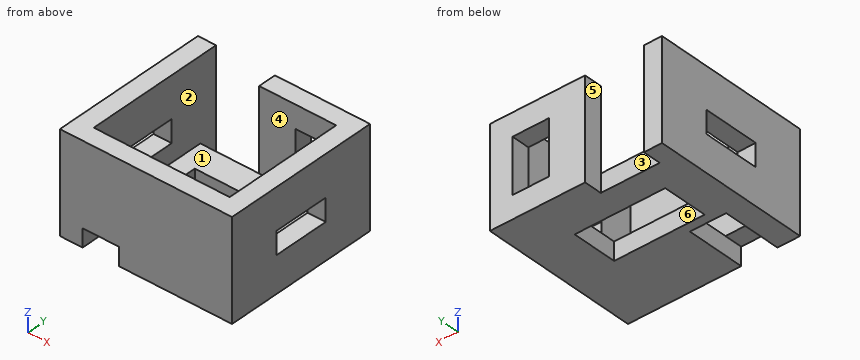
from build123d import *

# Parameters (mm, degrees)
F0_W     = 4
F0_H     = 4
F0_W_2   = 10
F0_H_2   = 5
F1_DEPTH = 2
F2_DEPTH = 11
F3_W     = 4
F3_H     = 6
F4_DEPTH = 2.9
F5_W     = 6.25
F5_H     = 2.5
F6_DEPTH = 20
F7_W     = 4
F7_H     = 2
F8_DEPTH = 2.8


with BuildPart() as f1:
    # F0 (on Top) → F1 (new body)
    with BuildSketch(Plane.XY):
        Polygon((-7.5, -6.75), (7.5, -6.75), (7.5, 6.75), (-1, 6.75), (-7.5, 6.75), align=None)
        with Locations((-5, -4.25)):
            Rectangle(F0_W, F0_H, mode=Mode.SUBTRACT)
        with Locations((-0.5, 1.25)):
            Rectangle(F0_W_2, F0_H_2, mode=Mode.SUBTRACT)
    extrude(amount=F1_DEPTH)

    # F0 (on Top) → F2 (join)
    with BuildSketch(Plane.XY):
        Polygon((7.5, 6.75), (7.5, -6.75), (-7.5, -6.75), (-7.5, 6.75), (-7.5, 8.75), (-9.5, 8.75), (-9.5, -8.75), (9.5, -8.75), (9.5, 8.75), (-1, 8.75), (-1, 6.75), align=None)
    extrude(amount=F2_DEPTH)

    # F3 (on face) → F4 (cut)
    with BuildSketch(Plane(origin=(0, 8.75, 0), x_dir=(-1, 0, 0), z_dir=(0, 1, 0))):
        with Locations((-5, 5.5)):
            Rectangle(F3_W, F3_H)
    extrude(amount=-F4_DEPTH, mode=Mode.SUBTRACT)

    # F5 (on face) → F6 (cut)
    with BuildSketch(Plane.YZ.offset(9.5)):
        with Locations((0, 5.25)):
            Rectangle(F5_W, F5_H)
    extrude(amount=-F6_DEPTH, mode=Mode.SUBTRACT)

    # F7 (on face) → F8 (cut)
    with BuildSketch(Plane.XZ.offset(8.75)):
        with Locations((-5, 1)):
            Rectangle(F7_W, F7_H)
    extrude(amount=-F8_DEPTH, mode=Mode.SUBTRACT)


solid = f1.part
Here's how the part is built. I have some questions about the finished solid (model axes, mm). Face numbers are marked on the shaded views. A direction names the side the tool comes from. Give positions to 0.01 mm unless a question says otherwise; leave off trailing zeros. Order: outer loops, then holes, each group sorted by start corner. A loop starts at its lowest first (then second) coordinate and runs counter-clockwise, first axis right, second up. Notation, with made-up numbers: (31.25, 32.5) -> (84.25, 32.5) arc R24 ccw to (84.25, 46.5) -> close; hole circle Ø11 at (53, 30). An arc over 180 degrees is marked (long way). One line per item, written item: value. Start each with the question number.
1. Imagine slicing it at D-D, the plane y = -1.5. List the corners of the cut face in (x, z) for me.
2. I need wall thicknesses on probe 1 along X at (y, z) = (-6.25, 4.25); probe 2 along Y at (x, z) = (2.25, 2.5); probe 3 along Y at (x, z) = (-4.5, 2.75). Which ranges of each line are inside material? Lowest first, please. Write a range as from..to.
3. Imagine slicing it at A-A, the plane y = -6. List the corners of the cut face in (x, z) for me, plus the area to 3 significant figures.
4. Imagine slicing it at C-C, the plane z = 6.75. List the corners of the cut face in (x, y) for me, plus the area to 3 significant figures.
5. For the marked faces 4, 5 and 6, which set-ups out of +Z, -Z, +X, -X, +Y, -Y let a thin tool reach every point of the face, with its end or its side?
6. Imagine slicing it at B-B, the plane x = 0. List the corners of the cut face in (y, z) for me.
7. Will these pins go through, and if not, where does the flat tip stop? pin 1 Ø5 at (x, y) = (-1.5, 4) entering from -Z; pin 2 Ø1 at (x, y) = (-4.5, -7.5) entering from -Z; pin 3 Ø7 at (x, y) = (2.5, -2.5) entering from +Z.
8. We'd pull the mould along Y, two halves only. Please class the marked faces 1, 2 and 3: released by +Y, released by -Y, zero draft, split by the parting line, or undercut.
Values follow:
1. outline: (-9.5, 0) -> (9.5, 0) -> (9.5, 4) -> (7.5, 4) -> (7.5, 2) -> (-7.5, 2) -> (-7.5, 4) -> (-9.5, 4) -> close; (-9.5, 6.5) -> (-7.5, 6.5) -> (-7.5, 11) -> (-9.5, 11) -> close; (7.5, 6.5) -> (9.5, 6.5) -> (9.5, 11) -> (7.5, 11) -> close
2. probe 1: x = -9.5..-7.5, 7.5..9.5
2. probe 2: y = -8.75..-6.75, 6.75..8.75
2. probe 3: y = -8.75..-6.75
3. outline: (-9.5, 0) -> (-7, 0) -> (-7, 2) -> (-7.5, 2) -> (-7.5, 11) -> (-9.5, 11) -> close; (-3, 0) -> (9.5, 0) -> (9.5, 11) -> (7.5, 11) -> (7.5, 2) -> (-3, 2) -> close
3. area: 66.0 mm2
4. outline: (-9.5, -8.75) -> (9.5, -8.75) -> (9.5, 8.75) -> (7, 8.75) -> (7, 6.75) -> (7.5, 6.75) -> (7.5, -6.75) -> (-7.5, -6.75) -> (-7.5, 8.75) -> (-9.5, 8.75) -> close; (-1, 6.75) -> (3, 6.75) -> (3, 8.75) -> (-1, 8.75) -> close
4. area: 109 mm2
5. face 4: +Z
5. face 5: +Z, -Z, +Y
5. face 6: +Z, -Z
6. outline: (-8.75, 0) -> (-1.25, 0) -> (-1.25, 2) -> (-6.75, 2) -> (-6.75, 11) -> (-8.75, 11) -> close; (3.75, 0) -> (8.75, 0) -> (8.75, 11) -> (6.75, 11) -> (6.75, 2) -> (3.75, 2) -> close
7. pin 1: stops at z = 0
7. pin 2: stops at z = 2
7. pin 3: stops at z = 2
8. face 1: undercut
8. face 2: zero draft
8. face 3: released by +Y
